Build history of the part. All positions in model axes, mm. A direction names the side the tool comes from. Round coordinates to 2 decimals unless told otherwise and drop trailing zeros. Write each loop counter-clockwise with the first axis right and the second up, starting at its lowest first coordinate (ties: lowest second). Pieces come first, ordered by that corner, then holes. Notation, with made-up numbers: (88, 77) -> (126, 77) arc R21 cw to (126, 85) -> close; hole circle Ø1 at (4.25, 89.5). An arc over 180 degrees is marked (long way). Answer as CSV lines item,"result".
from build123d import *

# Parameters (mm, degrees)
SKETCH1_R                  = 47.8
SKETCH1_R_2                = 41.5
CAP_BASE_DEPTH             = 15
SKETCH2_R                  = 47.8
CAP_TOP_DEPTH              = 10
SIDES_START                = 41.4
SIDES_DEPTH                = 6.5
SIDES_START_2              = -25
SIDES_TO_CAP_DEPTH         = 25
SKETCH5_R                  = 40.2
TRACKS_FOR_HOUSING_DEPTH   = 45
SKETCH6_R                  = 10.6
HOLE_FOR_GEAR_SHAFTS_DEPTH = 146.82002606
SKETCH9_R                  = 1.5
CUT_EXTRUDE2_DEPTH         = 10
CIRPATTERN1_COUNT          = 2
CIRPATTERN1_ANGLE          = 25
MIRROR2_COPY_1_SKETCH_R    = 1.5
MIRROR2_COPY_1_DEPTH       = 10
SKETCH10_R                 = 3.1
CUT_EXTRUDE3_DEPTH         = 2
CIRPATTERN2_COUNT          = 2
CIRPATTERN2_ANGLE          = 25
MIRROR3_COPY_1_SKETCH_R    = 3.1
MIRROR3_COPY_1_DEPTH       = 2


with BuildPart() as part:
    # Sketch1 → Cap base (new body)
    with BuildSketch(Plane(origin=(0, 0, 0), x_dir=(1, 0, 0), z_dir=(0, 1, 0))):
        with Locations(Location((0, 0, 0), (0, 0, 270))):
            Circle(SKETCH1_R)
        with Locations(Location((0, 0, 0), (0, 0, 270))):
            Circle(SKETCH1_R_2, mode=Mode.SUBTRACT)
    extrude(amount=CAP_BASE_DEPTH)

    # Sketch2 → Cap top (add)
    with BuildSketch(Plane(origin=(0, 15, 0), x_dir=(1, 0, 0), z_dir=(0, 1, 0))):
        with Locations(Location((0, 0, 0), (0, 0, 270))):
            Circle(SKETCH2_R)
    extrude(amount=CAP_TOP_DEPTH)

    # Sketch3 → Sides (add)
    with BuildSketch(Plane.XY.offset(SIDES_START)):
        with BuildLine():
            Line((-40, 59), (-40, 0))
            Line((-40, 0), (40, 0))
            Line((40, 0), (40, 59))
            ThreePointArc((40, 59), (0, 99), (-40, 59))
        make_face()
    sides = extrude(amount=SIDES_DEPTH)

    # Sketch4 → Sides to cap (add)
    with BuildSketch(Plane(origin=(0, 25, 0), x_dir=(1, 0, 0), z_dir=(0, 1, 0)).offset(SIDES_START_2)):
        with BuildLine():
            ThreePointArc((-23.893095237, -41.4), (-36.205132569, -31.209427673), (-44.469611721, -17.529792737))
            ThreePointArc((-44.469611721, -17.529792737), (-41.281194911, -29.286336098), (-40, -41.4))
            Line((-40, -41.4), (-23.893095237, -41.4))
        make_face()
        with BuildLine():
            Line((23.893095237, -41.4), (40, -41.4))
            ThreePointArc((40, -41.4), (41.281194911, -29.286336098), (44.469611721, -17.529792737))
            ThreePointArc((44.469611721, -17.529792737), (36.205132569, -31.209427673), (23.893095237, -41.4))
        make_face()
    sides_to_cap = extrude(amount=SIDES_TO_CAP_DEPTH)

    # Mirror1: Sides to cap across plane
    add(sides_to_cap.mirror(Plane.XY))

    # Mirror sides: Sides across plane
    add(sides.mirror(Plane.XY))

    # Sketch5 → Tracks for housing (cut)
    with BuildSketch(Plane(origin=(0, 0, 41.4), x_dir=(-1, 0, 0), z_dir=(0, 0, -1))):
        with Locations((0, 59)):
            Circle(SKETCH5_R)
    tracks_for_housing = extrude(amount=TRACKS_FOR_HOUSING_DEPTH, mode=Mode.SUBTRACT)

    # Mirror tracks: Tracks for housing across plane
    add(tracks_for_housing.mirror(Plane.XY), mode=Mode.SUBTRACT)

    # Sketch6 → Hole for gear shafts (cut, through all)
    with BuildSketch(Plane.XY.offset(47.9)):
        with Locations((0, 59)):
            Circle(SKETCH6_R)
    extrude(amount=-HOLE_FOR_GEAR_SHAFTS_DEPTH, mode=Mode.SUBTRACT)

    # Sketch9 → Cut-Extrude2 (cut)
    with BuildSketch(Plane(origin=(46.73476934, 0, -10.035005469), x_dir=(-0.20993735290442256, 0, -0.9777148397439225), z_dir=(0.9777148397439225, 0, -0.20993735290442256))):
        with Locations((0, 7.5)):
            Circle(SKETCH9_R)
    cut_extrude2 = extrude(amount=-CUT_EXTRUDE2_DEPTH, mode=Mode.SUBTRACT)

    # CirPattern1: Cut-Extrude2 ×2 about axis
    cirpattern1_axis = Axis((0, 15, 0), (0, -1, 0))
    for i in range(1, CIRPATTERN1_COUNT):
        add(cut_extrude2.rotate(cirpattern1_axis, i * CIRPATTERN1_ANGLE / (CIRPATTERN1_COUNT - 1)), mode=Mode.SUBTRACT)

    # Mirror2: Cut-Extrude2 across plane
    add(cut_extrude2.mirror(Plane(origin=(0, 0, 0), x_dir=(0, 0, 1), z_dir=(1, 0, 0))), mode=Mode.SUBTRACT)

    # Mirror2 copy 1 sketch → Mirror2 copy 1 (cut)
    with BuildSketch(Plane(origin=(-46.597061946, 0, 10.656163382), x_dir=(-0.2229322883235245, 0, -0.9748339319201179), z_dir=(-0.9748339319201179, 0, 0.2229322883235245))):
        with Locations((0, -7.5)):
            Circle(MIRROR2_COPY_1_SKETCH_R)
    extrude(amount=-MIRROR2_COPY_1_DEPTH, mode=Mode.SUBTRACT)

    # Sketch10 → Cut-Extrude3 (cut)
    with BuildSketch(Plane(origin=(46.73476934, 0, -10.035005469), x_dir=(-0.20993735290442256, 0, -0.9777148397439225), z_dir=(0.9777148397439225, 0, -0.20993735290442256))):
        with Locations((0, 7.5)):
            Circle(SKETCH10_R)
    cut_extrude3 = extrude(amount=-CUT_EXTRUDE3_DEPTH, mode=Mode.SUBTRACT)

    # CirPattern2: Cut-Extrude3 ×2 about axis
    cirpattern2_axis = Axis((0, 15, 0), (0, -1, 0))
    for i in range(1, CIRPATTERN2_COUNT):
        add(cut_extrude3.rotate(cirpattern2_axis, i * CIRPATTERN2_ANGLE / (CIRPATTERN2_COUNT - 1)), mode=Mode.SUBTRACT)

    # Mirror3: Cut-Extrude3 across plane
    add(cut_extrude3.mirror(Plane(origin=(0, 0, 0), x_dir=(0, 0, 1), z_dir=(1, 0, 0))), mode=Mode.SUBTRACT)

    # Mirror3 copy 1 sketch → Mirror3 copy 1 (cut)
    with BuildSketch(Plane(origin=(-46.597061946, 0, 10.656163382), x_dir=(-0.22293228832352457, 0, -0.9748339319201178), z_dir=(-0.9748339319201178, 0, 0.22293228832352457))):
        with Locations((0, -7.5)):
            Circle(MIRROR3_COPY_1_SKETCH_R)
    extrude(amount=-MIRROR3_COPY_1_DEPTH, mode=Mode.SUBTRACT)


solid = part.part
1. Probe line 1 along Y through (x, z) = (0, 46.25); line 2 along Z through (x, y) = (-14.5, 53); line 3 along Y through (x, z) = (34.5, -22.5). List the from-to ranges inside material, lowest first.
Results found:
line 1,"y = 0 to 48.4, 69.6 to 99"
line 2,"z = -47.9 to -41.4, 41.4 to 47.9"
line 3,"y = 15 to 25"
2. Cut at A-A, the plane y = 35. Write the cut outline in (x, z), then the cut area to 3 significant figures.
Results found:
outline,"(-40, -47.9) -> (40, -47.9) -> (40, -41.4) -> (-40, -41.4) -> close; (-40, 41.4) -> (40, 41.4) -> (40, 47.9) -> (-40, 47.9) -> close"
area,"1,040 mm2"
3. Cut at B-B, the plane x = 0. Write the cut outline in (y, z), then the cut area to 3 significant figures.
Results found:
outline,"(0, -47.9) -> (48.4, -47.9) -> (48.4, -41.4) -> (18.8, -41.4) -> (18.8, 41.4) -> (48.4, 41.4) -> (48.4, 47.9) -> (0, 47.9) -> (0, 41.4) -> (15, 41.4) -> (15, -41.4) -> (0, -41.4) -> close; (69.6, -47.9) -> (99, -47.9) -> (99, -41.4) -> (69.6, -41.4) -> close; (69.6, 41.4) -> (99, 41.4) -> (99, 47.9) -> (69.6, 47.9) -> close"
area,"1,330 mm2"
4. Drop flat-ended pins along their axis: pin 1 Ø1 at (x, z) = (-26.5, -10) entering from -Y; pin 2 Ø5 at (y, z) = (40.5, 45) entering from +X; pin 3 Ø13 at (x, z) = (36, 13.5) entering from +Y. Give the stop position or say it passes through.
Results found:
pin 1,"stops at y = 15"
pin 2,"stops at x = 40"
pin 3,"stops at y = 25"
5. Cut at C-C, the plane z = 0. Write the cut outline in (x, y), then the cut area to 3 significant figures.
Results found:
outline,"(-47.8, 0) -> (-41.5, 0) -> (-41.5, 15) -> (41.5, 15) -> (41.5, 0) -> (47.8, 0) -> (47.8, 25) -> (21.45, 25) arc R40.2 cw to (-21.45, 25) -> (-47.8, 25) -> close"
area,"965 mm2"
6. Which spindle directions (+Z, -Z, +X, -X, +Y, -Y) get a long thin tool onto all of the face, cutting with end or side? Do faces 5 (the flat face through (-40, 30, -45)), 6 (the flat face through (32, 25, -1)), 7 (the cylindrical face through (-42.495, 8.964, 10.052)). Say none if no direction does.
Results found:
face 5,"-Z, -X, +Y, -Y"
face 6,"+X, -X, +Y"
face 7,"none"
7. Mould opens along Z. For faces 1 (the cylindrical face through (41.25, 12.32, -29.45)), 2 (the flat face through (0, 8, 41.4)), 3 (the flat face through (-40, 30, 45)), 4 (the cylindrical face through (-45.15, 8.43, -12.72)) say: +Z half, -Z half, draft (parallel to the pull), parting line (faces both ways), or undercut.
Results found:
face 1,"-Z half"
face 2,"undercut"
face 3,"draft"
face 4,"undercut"
8. Cut at D-D, the plane y = 62.5. Write the cut outline in (x, z), then the cut area to 3 significant figures.
Results found:
outline,"(-39.85, -47.9) -> (-10.01, -47.9) -> (-10.01, -41.4) -> (-39.85, -41.4) -> close; (-39.85, 41.4) -> (-10.01, 41.4) -> (-10.01, 47.9) -> (-39.85, 47.9) -> close; (10.01, -47.9) -> (39.85, -47.9) -> (39.85, -41.4) -> (10.01, -41.4) -> close; (10.01, 41.4) -> (39.85, 41.4) -> (39.85, 47.9) -> (10.01, 47.9) -> close"
area,"776 mm2"
